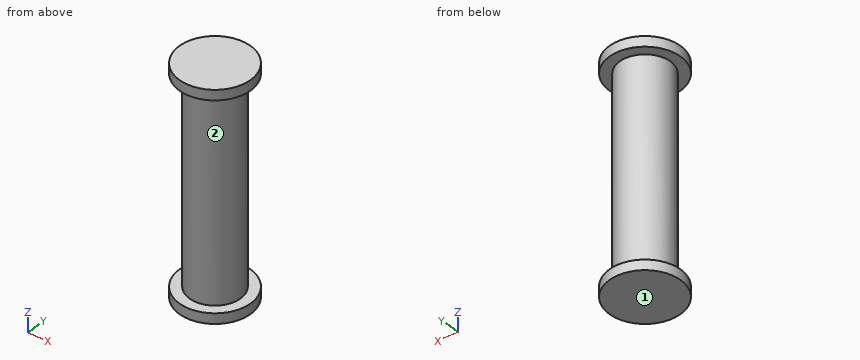
from build123d import *

# Parameters (mm, degrees)
SKETCH_1_R        = 5
EXTRUDE_1_DEPTH   = 42
SKETCH_3_R        = 7
SKETCH_3_R_2      = 5
EXTRUDE_2_DEPTH   = 2
SKETCH_4_R        = 7
SKETCH_4_R_2      = 5
EXTRUDE_4_DEPTH   = 2
SKETCH_5_R        = 5
EXTRUDE_2_2_DEPTH = 2


with BuildPart() as part:
    # 草图1 → 凸台-拉伸1 (new body)
    with BuildSketch(Plane.XY):
        with Locations(Location((0, 0, 0), (0, 0, 180))):
            Circle(SKETCH_1_R)
    extrude(amount=EXTRUDE_1_DEPTH)

    # 草图3 → Extrude 2 (add)
    with BuildSketch(Plane(origin=(0, 0, 0), x_dir=(-1, 0, 0), z_dir=(0, 0, -1))):
        Circle(SKETCH_3_R)
        Circle(SKETCH_3_R_2, mode=Mode.SUBTRACT)
    extrude(amount=-EXTRUDE_2_DEPTH)



with BuildPart() as body_2:
    # 草图4 → 拉伸-薄壁4 (new body)
    with BuildSketch(Plane.XY.offset(42)):
        Circle(SKETCH_4_R)
        Circle(SKETCH_4_R_2, mode=Mode.SUBTRACT)
    extrude(amount=EXTRUDE_4_DEPTH)


with BuildPart() as part_1:
    add(part.part)

    add(body_2.part)  # Extrude 2 2 merges body 2
    # 草图5 → Extrude 2 2 (add)
    with BuildSketch(Plane.XY.offset(42)):
        with Locations(Location((0, 0, 0), (0, 0, 180))):
            Circle(SKETCH_5_R)
    extrude(amount=EXTRUDE_2_2_DEPTH)


solid = part_1.part
Geometry: final body of the model. Coordinates: model frame, mm. Face numbers are marked on the shaded views. Coordinates: 2 decimals unless noted, no trailing zeros. Write each loop counter-clockwise with the first axis right and the second up, starting at its lowest first coordinate (ties: lowest second). Pieces come first, ordered by that corner, then holes. Notation, with made-up numbers: (69, 20) - (125, 20) arc R16 cw to (125, 26) - close; hole circle Ø6 at (-31, 35.5). An arc over 180 degrees is marked (long way). Return JSON: item names as keys, results as strings.
Item 1: Pull-direction query (Y, two-part tool) for the marked faces 1 and 2; classes: +Y half, -Y half, draft (parallel to the pull), parting line (faces both ways), or undercut.
Completed:
{"face 1": "draft", "face 2": "parting line"}
Item 2: Pin query (flat end, axial travel): pin 1 Ø6 at (x, z) = (-0.5, 34.5) entering from +Y; pin 2 Ø6 at (y, z) = (-1, 36) entering from +X; pin 3 Ø1 at (x, z) = (4.5, 5) entering from -Y. Return the tip coordinate at first contact, or that it passes through.
Completed:
{"pin 1": "stops at y = 5", "pin 2": "stops at x = 5", "pin 3": "stops at y = -3"}
Item 3: Section query A-A (x = 0). Output: boundary loops of the cut face in (y, z), and give its area (3 significant figures).
Completed:
{"outline": "(-7, 0) - (7, 0) - (7, 2) - (5, 2) - (5, 42) - (7, 42) - (7, 44) - (-7, 44) - (-7, 42) - (-5, 42) - (-5, 2) - (-7, 2) - close", "area": "456 mm2"}
Item 4: Section query C-C (z = 35.5). Output: boundary loops of the cut face in (x, y), and give its area (3 significant figures).
Completed:
{"outline": "circle Ø10 at (0, 0)", "area": "78.5 mm2"}
Item 5: Line query: L1, parallel to Z at x = -0.5, y = -5.5; L2, parallel to X at y = 0.25, z = 34.5. Output: solid intervals per line, ascending.
Completed:
{"L1": "z = 0 to 2, 42 to 44", "L2": "x = -4.99 to 4.99"}
